For this review, take the finished solid that the model builds, in its own axes (mm). A direction names the side the tool comes from. Give positions to 0.01 mm unless a question says otherwise; leave off trailing zeros. Loops run counter-clockwise (first coordinate to the right, second up) from the corner with the lowest first, then second, coordinate; pieces in that order, holes last.
```python
from build123d import *

# Parameters (mm, degrees)
F1_DEPTH = 25.4


with BuildPart() as f1:
    # F0 (on Front) → F1 (new body)
    with BuildSketch(Plane.XZ):
        Polygon((-50.8, 0), (0, 50.8), (0, 76.2), (-76.2, 0), align=None)
        with BuildLine():
            Line((0, 76.2), (0, 50.8))
            ThreePointArc((0, 50.8), (35.921024, 35.921024), (50.8, 0))
            Line((50.8, 0), (76.2, 0))
            ThreePointArc((76.2, 0), (53.881537, 53.881537), (0, 76.2))
        make_face()
    extrude(amount=F1_DEPTH)


solid = f1.part
```
Item 1: Take a section at D-D on z = 40. Give the boundary of the cut face in (x, y).
Answer:
outline: (-36.2, -25.4) - (-10.8, -25.4) - (-10.8, 0) - (-36.2, 0) - close; (31.32, -25.4) - (64.86, -25.4) - (64.86, 0) - (31.32, 0) - close
Item 2: Take a section at C-C on x = -18.5. Give the boundary of the cut face in (y, z).
Answer:
outline: (-25.4, 32.3) - (0, 32.3) - (0, 57.7) - (-25.4, 57.7) - close
Item 3: Clearance check with flat-ended pins moving along their axes: pin 1 Ø4 at (x, y) = (32.5, -17) entering from +Z; pin 2 Ø6 at (y, z) = (-6, 44) entering from -X; pin 3 Ø3 at (y, z) = (-15, 10.5) entering from -X. State where each tip first meets the part, or that it passes through.
Answer:
pin 1: stops at z = 69.83
pin 2: stops at x = -35.2
pin 3: stops at x = -67.2
Item 4: Take a section at B-B on y = -20.5. Give the boundary of the cut face in (x, z).
Answer:
outline: (-76.2, 0) - (-50.8, 0) - (0, 50.8) arc R50.8 cw to (50.8, 0) - (76.2, 0) arc R76.2 ccw to (0, 76.2) - close
Item 5: Take a section at A-A on z = 26.5. Give the boundary of the cut face in (x, y).
Answer:
outline: (-49.7, -25.4) - (-24.3, -25.4) - (-24.3, 0) - (-49.7, 0) - close; (43.34, -25.4) - (71.44, -25.4) - (71.44, 0) - (43.34, 0) - close
Item 6: The part is to be moulded in two halves that separate along X. For faces 3 (the flat face through (22, 0, 52)), 4 (the cylindrical face through (54.471, -12.522, 53.286)), 5 (the cylindrical face through (35.524, -12.522, 36.314)), say which applies: released by +X, released by -X, zero draft, split by the parting line, or undercut.
Answer:
face 3: zero draft
face 4: released by +X
face 5: undercut
Item 7: Tool access review of faces 1 (the flat face through (-64, -13, 0)), 2 (the flat face through (-25.8, -12.5, 25)): name each direction out of +Z, -Z, +X, -X, +Y, -Y from which nothing blocks a thin tool from reaching the whole face with its end or side.
Answer:
face 1: -Z, +X, -X, +Y, -Y
face 2: -Z, +Y, -Y
Item 8: For L1, parallel to X at y = -6.25, z = 38; L2, parallel to X at y = -15, z = 39; L3, parallel to X at y = -1.5, z = 58.5, list the stretches that pass through material, from the lowest coordinate up.
Answer:
L1: x = -38.2 to -12.8, 33.71 to 66.05
L2: x = -37.2 to -11.8, 32.55 to 65.46
L3: x = -17.7 to 48.83
